Geometry check sheet. Reference: the model listing, model coordinates, mm. A direction names the side the tool comes from. Coordinates: 2 decimals unless noted, no trailing zeros. Order: outer loops, then holes, each group sorted by start corner. A loop starts at its lowest first (then second) coordinate and runs counter-clockwise, first axis right, second up. Notation, with made-up numbers: (49, 14) - (79, 14) arc R30 ccw to (79, 45) - close; hole circle Ø6 at (11.25, 69). An arc over 180 degrees is marked (long way). Return JSON: item names as keys, results as strings. Group by question number.
Item 1: Draft check along Z on faces 1 (the flat face through (22, 163.6, 83)), 2 (the flat face through (22, 81, 0)), 3 (the cylindrical face through (5.07, 1.02, 170.18)). Enter one of: pulls with the +Z half, pulls with the -Z half, needs draft (parallel to the pull), parting line crosses it, or undercut.
Item 2: Section check B-B on y = 119.5. Enter the section's corners in (x, z), then the cut area to 3 significant figures.
Item 3: Scan lines: probe 1 along Z at (x, y) = (4.5, 108.5); probe 2 along Z at (x, y) = (5, 0.6). Record each from-to range of solid material in increasing order.
Item 4: Tool access check on faces 4 (the flat face through (45, 81, 85)), 5 (the flat face through (5, 2, 170)). Record the directions out of +Z, -Z, +X, -X, +Y, -Y that give a thin tool (end or side, any length) a straight path to the whole face; none if there is none.
Item 5: Section check C-C on x = 16.5. Enter the section's corners in (y, z), then the cut area to 3 significant figures.
Item 6: Gauge pin test, flat ends, axial feed: pin 1 (6 mm diameter, centred on x = 5, z = 172.68, fed in from +Y); pin 2 (4 mm diameter, centred on x = 7, y = 141, fed in from +Z); pin 3 (1 mm diameter, centred on y = 1.5, z = 170, fed in from +X). Record the tip position at first contact, or that the pin passes through.
from build123d import *

# Parameters (mm, degrees)
SKETCH_1_W            = 45
SKETCH_1_H            = 168
EXTRUDE_1_DEPTH       = 163.6
SKETCH_2_W            = 10
SKETCH_2_H            = 6
EXTRUDE_2_DEPTH       = 2
F_5_0MM_1_D           = 5
F_5_0MM_1_CSINK_D     = 5.05
F_5_0MM_1_CSINK_ANGLE = 100


with BuildPart() as part:
    # 草图1 → 凸台-拉伸1 (new body)
    with BuildSketch(Plane(origin=(0, 0, 0), x_dir=(1, 0, 0), z_dir=(0, 1, 0))):
        with Locations((22.5, -84)):
            Rectangle(SKETCH_1_W, SKETCH_1_H)
    extrude(amount=EXTRUDE_1_DEPTH)

    # 草图2 → 凸台-拉伸2 (add)
    with BuildSketch(Plane.XZ):
        with Locations((5, 171)):
            Rectangle(SKETCH_2_W, SKETCH_2_H)
    extrude(amount=-EXTRUDE_2_DEPTH)

    # Ø5.0mm 暗销孔1 (through all)
    with Locations(Plane(origin=(0, 0, 0), x_dir=(-1, 0, 0), z_dir=(0, -1, 0))):
        with Locations((-5, -172.677656)):
            CounterSinkHole(F_5_0MM_1_D / 2, F_5_0MM_1_CSINK_D / 2, counter_sink_angle=F_5_0MM_1_CSINK_ANGLE)


solid = part.part
Computed:
{
 "1": {"face 1": "needs draft", "face 2": "pulls with the -Z half", "face 3": "undercut"},
 "2": {"outline": "(0, 0) - (45, 0) - (45, 168) - (0, 168) - close", "area": "7,560 mm²"},
 "3": {"probe 1": "z = 0 to 168", "probe 2": "z = 0 to 170.18"},
 "4": {"face 4": "+Z, -Z, +X, +Y, -Y", "face 5": "+Z, +X, -X, +Y"},
 "5": {"outline": "(0, 0) - (163.6, 0) - (163.6, 168) - (0, 168) - close", "area": "27,500 mm²"},
 "6": {"pin 1": "stops at y = 2", "pin 2": "stops at z = 168", "pin 3": "stops at x = 10"}
}
